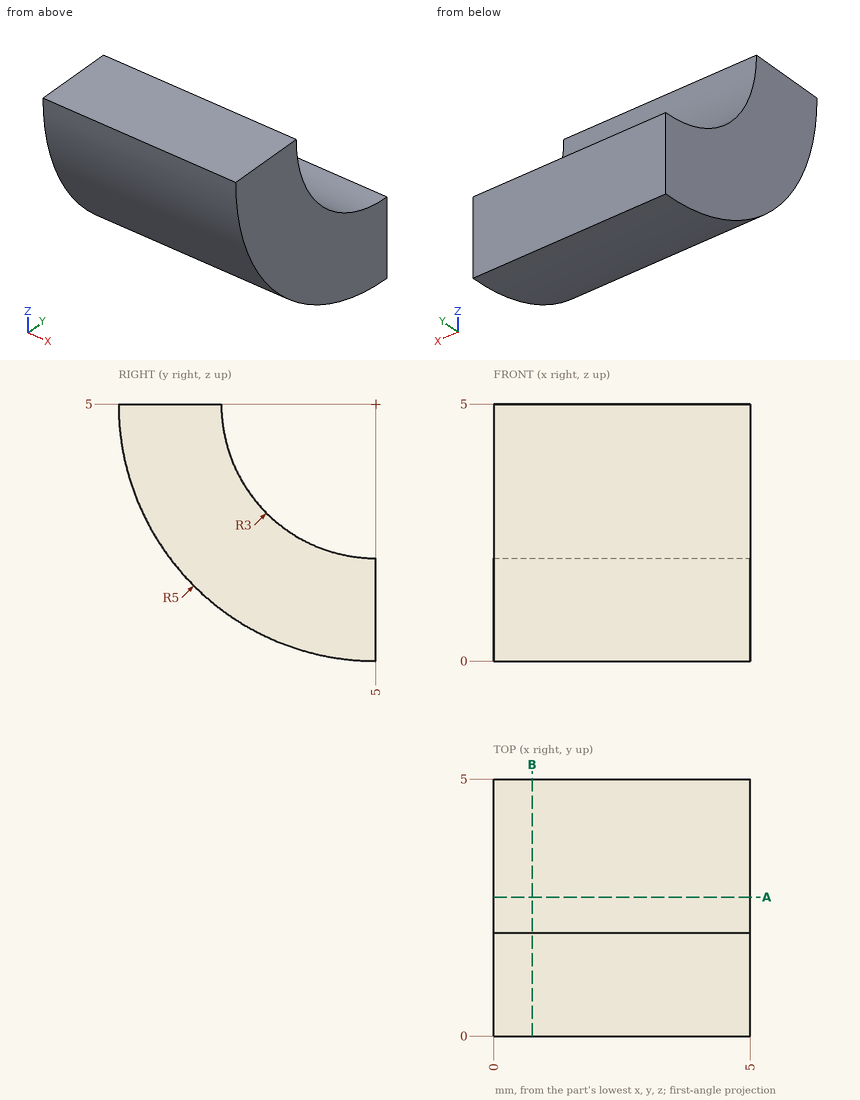
Study the drawing (mm; zero at the part's minimum x, y, z) and answer. Round coordinates to 2 decimals unless told otherwise and drop trailing zeros. Write each loop counter-clockwise with the first axis right and the second up, starting at its lowest first coordinate (ties: lowest second). Pieces come first, ordered by that corner, then holes.
1) Straight lines are drawn through the part: line 1 (Y direction, x = 4.55, z = 2.8); line 2 (Z direction, x = 0.5, y = 2.25); line 3 (Z direction, x = 0.5, y = 4.65). For each, find the intervals that lie inside material, in ascending order.
2) Given pin 1 Ø1.5 at (x, y) = (1, 1.5) entering from -Z, flat-ended and moving along its own axis, determine where the tip first touches the part or whether it passes through.
3) A cutting plane is placed at A-A (y = 2.7). Give the vertices of the cut face in (x, z).
4) A cutting plane is placed at B-B (x = 0.75). Give the vertices of the cut face in (y, z), plus the area to 3 significant figures.
Completed:
1. line 1: y = 0.51 to 2.96
1. line 2: z = 0.82 to 3.8
1. line 3: z = 0.01 to 2.02
2. pin 1: stops at z = 0.82
3. outline: (0, 0.56) - (5, 0.56) - (5, 3.07) - (0, 3.07) - close
4. outline: (0, 5) arc R5 ccw to (5, 0) - (5, 2) arc R3 cw to (2, 5) - close
4. area: 12.6 mm2
